The listing builds one solid part. Answer for the finished solid, in the listing's coordinates (mm). Face numbers are marked on the shaded views. A direction names the side the tool comes from. Coordinates: 2 decimals unless noted, no trailing zeros. Loops run counter-clockwise (first coordinate to the right, second up) from the corner with the lowest first, then second, coordinate; pieces in that order, holes last. Notation, with made-up numbers: (41, 79.25) -> (88, 79.25) arc R25 ccw to (88, 114.25) -> close; hole circle Ø7 at (-24.5, -13). An arc over 180 degrees is marked (long way). Answer in a Markdown table with one row per item.
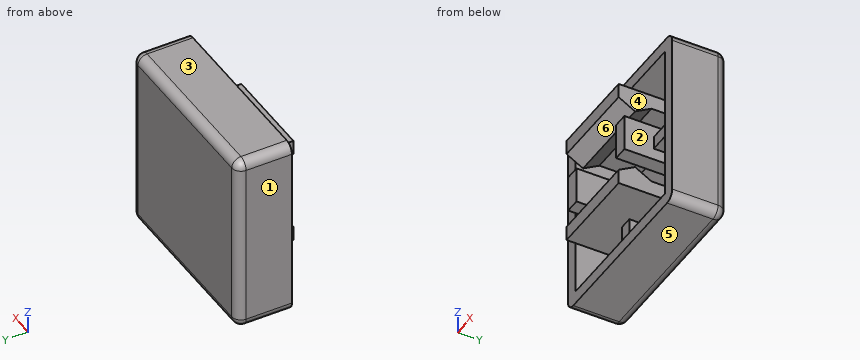
```python
from build123d import *

# Parameters (mm, degrees)
SKETCH1_W             = 10
SKETCH1_H             = 10
BOSS_EXTRUDE2_DEPTH   = 3
SHELL2_T              = -0.7
FILLET2_R             = 0.5
BOSS_EXTRUDE3_DEPTH   = 2.5
BOSS_EXTRUDE3_2_DEPTH = 2.5
SKETCH6_W             = 0.8
SKETCH6_H             = 3.8
BOSS_EXTRUDE4_DEPTH   = 1
SKETCH7_W             = 1.5
SKETCH7_H             = 2.2
BOSS_EXTRUDE5_DEPTH   = 0.35
SKETCH9_W             = 1.8
SKETCH9_H             = 2.2
BOSS_EXTRUDE6_DEPTH   = 0.35


with BuildPart() as part:
    # Sketch1 → Boss-Extrude2 (new body)
    with BuildSketch(Plane(origin=(0, 0, 0), x_dir=(1, 0, 0), z_dir=(0, 1, 0))):
        Rectangle(SKETCH1_W, SKETCH1_H)
    extrude(amount=-BOSS_EXTRUDE2_DEPTH)

    # Shell2
    shell2_openings = [part.faces().sort_by_distance(p)[0] for p in [
        (0, -3, 0),
    ]]
    offset(amount=SHELL2_T, openings=shell2_openings, kind=Kind.INTERSECTION)

    # Fillet2
    fillet2_edges = [part.edges().sort_by_distance(p)[0] for p in [
        (0, 0, 5),
        (-5, 0, 0),
        (0, 0, -5),
        (5, 0, 0),
        (5, -1.5, 5),
        (-5, -1.5, 5),
        (-5, -1.5, -5),
        (5, -1.5, -5),
    ]]
    fillet(fillet2_edges, radius=FILLET2_R)

    # Sketch6 → Boss-Extrude4 (add, symmetric)
    with BuildSketch(Plane.XY):
        with Locations((2.3, -2.4)):
            Rectangle(SKETCH6_W, SKETCH6_H)
        with Locations((-2.3, -2.4)):
            Rectangle(SKETCH6_W, SKETCH6_H)
    extrude(amount=BOSS_EXTRUDE4_DEPTH, both=True)



with BuildPart() as body_2:
    # Sketch5 → Boss-Extrude3 (new body, symmetric)
    with BuildSketch(Plane(origin=(0, 0, 0), x_dir=(0, 0, -1), z_dir=(1, 0, 0))):
        Polygon((3, -0.5), (3, -4.5), (2.2, -4.5), (1.683643362, -3.605644068), (2.2, -2.711288136), (2.2, -0.5), align=None)
    extrude(amount=BOSS_EXTRUDE3_DEPTH, both=True)


with BuildPart() as body_3:
    # Sketch5 → Boss-Extrude3 2 (new body, symmetric)
    with BuildSketch(Plane(origin=(0, 0, 0), x_dir=(0, 0, -1), z_dir=(1, 0, 0))):
        Polygon((-2.2, -0.5), (-3, -0.5), (-3, -4.5), (-2.2, -4.5), (-1.683643362, -3.605644068), (-2.2, -2.711288136), align=None)
    extrude(amount=BOSS_EXTRUDE3_2_DEPTH, both=True)


with BuildPart() as part_1:
    add(part.part)

    add(body_2.part)  # Boss-Extrude5 merges body 2

    add(body_3.part)  # Boss-Extrude5 merges body 3
    # Sketch7 → Boss-Extrude5 (add, symmetric)
    with BuildSketch(Plane(origin=(0, 0, 0), x_dir=(0, 0, -1), z_dir=(1, 0, 0))):
        with Locations((-3.75, -1.6)):
            Rectangle(SKETCH7_W, SKETCH7_H)
        with Locations((3.75, -1.6)):
            Rectangle(SKETCH7_W, SKETCH7_H)
    extrude(amount=BOSS_EXTRUDE5_DEPTH, both=True)

    # Sketch9 → Boss-Extrude6 (add, symmetric)
    with BuildSketch(Plane.XY):
        with Locations((-3.6, -1.6)):
            Rectangle(SKETCH9_W, SKETCH9_H)
        with Locations((3.6, -1.6)):
            Rectangle(SKETCH9_W, SKETCH9_H)
    extrude(amount=BOSS_EXTRUDE6_DEPTH, both=True)


solid = part_1.part
```
Item 1: A cutting plane is placed at A-A, the plane z = 2.5. Determine the outline of the cut face in (x, y).
Findings below:
| item | result |
|---|---|
| outline | (-5, -3) -> (-4.3, -3) -> (-4.3, -0.7) -> (-2.5, -0.7) -> (-2.5, -4.5) -> (2.5, -4.5) -> (2.5, -0.7) -> (4.3, -0.7) -> (4.3, -3) -> (5, -3) -> (5, -0.5) arc R0.5 ccw to (4.5, 0) -> (-4.5, 0) arc R0.5 ccw to (-5, -0.5) -> close |
Item 2: Determine the mould class of the marked faces 1, 2 and 3 for opening direction X: +X half, -X half, draft (parallel to the pull), parting line (faces both ways), or undercut.
Findings below:
| item | result |
|---|---|
| face 1 | -X half |
| face 2 | undercut |
| face 3 | draft |
Item 3: A flat-ended cylindrical pin translates along its axis: pin 1 Ø2 at (x, z) = (-4, 0) entering from -Y. Find the tip coordinate at first contact, or state that the pin passes through.
Findings below:
| item | result |
|---|---|
| pin 1 | stops at y = -3 |
Item 4: A cutting plane is placed at C-C, the plane y = -4.1. Determine the outline of the cut face in (x, z), plus the area to 3 significant figures.
Findings below:
| item | result |
|---|---|
| outline | (-2.7, -1) -> (-1.9, -1) -> (-1.9, 1) -> (-2.7, 1) -> close; (-2.5, -3) -> (2.5, -3) -> (2.5, -1.97) -> (-2.5, -1.97) -> close; (-2.5, 1.97) -> (2.5, 1.97) -> (2.5, 3) -> (-2.5, 3) -> close; (1.9, -1) -> (2.7, -1) -> (2.7, 1) -> (1.9, 1) -> close |
| area | 13.5 mm2 |
Item 5: A tool of negligible diameter and unlimited length cuts with its end or side. For the marked faces 4, 5 and 6, from which of +Z, -Z, +X, -X, +Y, -Y can it reach the whole face along a straight path? Write none if from no direction.
Findings below:
| item | result |
|---|---|
| face 4 | -Y |
| face 5 | -Z, +X, -X, +Y, -Y |
| face 6 | +X, -X, -Y |
Item 6: Find the intervals of material crossed by probe 1 along Z at (x, y) = (-2, -1); probe 2 along X at (y, z) = (-1.15, 2.5); probe 3 along Z at (x, y) = (-0.5, -2.3), in increasing order.
Findings below:
| item | result |
|---|---|
| probe 1 | z = -5 to -4.3, -3 to -2.2, -1 to 1, 2.2 to 3, 4.3 to 5 |
| probe 2 | x = -5 to -4.3, -2.5 to 2.5, 4.3 to 5 |
| probe 3 | z = -5 to -4.3, -3 to -2.2, 2.2 to 3, 4.3 to 5 |
Item 7: A cutting plane is placed at D-D, the plane z = 0. Determine the outline of the cut face in (x, y).
Findings below:
| item | result |
|---|---|
| outline | (-5, -3) -> (-4.3, -3) -> (-4.3, -2.7) -> (-2.7, -2.7) -> (-2.7, -4.3) -> (-1.9, -4.3) -> (-1.9, -0.7) -> (1.9, -0.7) -> (1.9, -4.3) -> (2.7, -4.3) -> (2.7, -2.7) -> (4.3, -2.7) -> (4.3, -3) -> (5, -3) -> (5, -0.5) arc R0.5 ccw to (4.5, 0) -> (-4.5, 0) arc R0.5 ccw to (-5, -0.5) -> close |
Item 8: A cutting plane is placed at B-B, the plane x = -1.75. Determine the outline of the cut face in (y, z).
Findings below:
| item | result |
|---|---|
| outline | (-4.5, -3) -> (-0.7, -3) -> (-0.7, -4.3) -> (-3, -4.3) -> (-3, -5) -> (-0.5, -5) arc R0.5 ccw to (0, -4.5) -> (0, 4.5) arc R0.5 ccw to (-0.5, 5) -> (-3, 5) -> (-3, 4.3) -> (-0.7, 4.3) -> (-0.7, 3) -> (-4.5, 3) -> (-4.5, 2.2) -> (-3.61, 1.68) -> (-2.71, 2.2) -> (-0.7, 2.2) -> (-0.7, -2.2) -> (-2.71, -2.2) -> (-3.61, -1.68) -> (-4.5, -2.2) -> close |
